Geometry check sheet. Reference: the model listing, model coordinates, mm. A direction names the side the tool comes from. Coordinates: 2 decimals unless noted, no trailing zeros. Write each loop counter-clockwise with the first axis right and the second up, starting at its lowest first coordinate (ties: lowest second). Pieces come first, ordered by that corner, then holes. Notation, with made-up numbers: (73, 87) -> (123, 87) arc R34 cw to (123, 124) -> close; hole circle Ø3 at (74, -4). An arc over 180 degrees is marked (long way). One line per question, with ' | ' between items.
from build123d import *

# Parameters (mm, degrees)
F0_R     = 19.05
F1_DEPTH = 2.54
F2_R     = 6.35
F3_DEPTH = 20.32
F5_R     = 19.05
F6_DEPTH = 30.48
F6_TAPER = 32


with BuildPart() as f1:
    # F0 (on Front) → F1 (new body)
    with BuildSketch(Plane.XZ):
        Circle(F0_R)
    extrude(amount=F1_DEPTH)

    # F2 (on face) → F3 (join)
    with BuildSketch(Plane.XZ.offset(2.54)):
        Circle(F2_R)
    extrude(amount=F3_DEPTH)

    # F5 (on offset) → F6 (join)
    with BuildSketch(Plane(origin=(0, -22.86, 0), x_dir=(-1, 0, 0), z_dir=(0, 1, 0))):
        Circle(F5_R)
    extrude(amount=-F6_DEPTH, taper=F6_TAPER)


solid = f1.part
1. Cross-section at B-B on y = -32.5. Record the boundary of the cut face in (x, z).
Worked answers:
outline: circle Ø26.05 at (0, 0)
2. Tool access check on faces 1 (the face through (5, -22.86, 5)), 2 (the face through (1.6, -41.7, -7.1)). Record the directions out of +Z, -Z, +X, -X, +Y, -Y that give a thin tool (end or side, any length) a straight path to the whole face; none if there is none.
Worked answers:
face 1: none | face 2: -Y
3. Cross-section at A-A on y = -3.5. Record the boundary of the cut face in (x, z).
Worked answers:
outline: circle Ø12.7 at (0, 0)
4. Material ranges on line 1 (Y direction, x = 16, z = -9); line 2 (Y direction, x = -8, z = -0.5); line 3 (X direction, y = -5, z = -4), recorded low to high. Write a range as from..to.
Worked answers:
line 1: -23.97..-22.86, -2.54..0 | line 2: -40.52..-22.86, -2.54..0 | line 3: -4.93..4.93
5. Go/stop test with flat-tipped pins: P1, Ø5, axis at x = 0.5, z = -7, coming from the -Y side; P2, Ø1.5, axis at y = -26, z = -3, coming from the +X side; P3, Ø1.5, axis at x = -9.5, z = 15, coming from the -Y side. Record where each tip stops, or that it passes through.
Worked answers:
P1: y = -46.12 | P2: x = 17.31 | P3: y = -26.13
6. Mould release check, pull along Y, two halves, no side actions. Record for faces 3 (the face through (-1.38, -12.56, -6.2)), 4 (the face through (0, 0, 0)), 5 (the face through (-15.12, -1.25, -11.59)): released by +Y, released by -Y, zero draft, split by the parting line, or undercut.
Worked answers:
face 3: undercut | face 4: released by +Y | face 5: zero draft
